Design review of the part built by this model. Coordinates are the model's own, in mm. A direction names the side the tool comes from. Coordinates: 2 decimals unless noted, no trailing zeros. Loops run counter-clockwise (first coordinate to the right, second up) from the corner with the lowest first, then second, coordinate; pieces in that order, holes last. Notation, with made-up numbers: (83, 30.25) -> (87, 30.25) arc R24 ccw to (87, 61.25) -> close; hole circle Ø9 at (24, -19). An arc over 180 degrees is marked (long way). Use CSV: the item, a comma, the result in double quotes.
```python
from build123d import *

# Parameters (mm, degrees)
SKETCH1_R           = 23
SKETCH1_R_2         = 0.725
BOSS_EXTRUDE1_DEPTH = 5
SKETCH2_W           = 4.5
SKETCH2_H           = 3.9
SKETCH2_W_2         = 3.9
SKETCH2_H_2         = 4.5
CUT_EXTRUDE1_DEPTH  = 6
SKETCH3_W           = 7
SKETCH3_H           = 4
SKETCH3_W_2         = 4
SKETCH3_H_2         = 7
CUT_EXTRUDE2_DEPTH  = 6


with BuildPart() as part:
    # Sketch1 → Boss-Extrude1 (new body)
    with BuildSketch(Plane.XY):
        Circle(SKETCH1_R)
        Circle(SKETCH1_R_2, mode=Mode.SUBTRACT)
    extrude(amount=BOSS_EXTRUDE1_DEPTH)

    # Sketch2 → Cut-Extrude1 (cut, through all)
    with BuildSketch(Plane(origin=(0, 0, 0), x_dir=(-1, 0, 0), z_dir=(0, 0, -1))):
        with Locations((9.999907629, 0.148804685)):
            Rectangle(SKETCH2_W, SKETCH2_H)
        with Locations((-0.147804685, 9.998907629)):
            Rectangle(SKETCH2_W_2, SKETCH2_H_2)
        with Locations((0.149804685, -9.998907629)):
            Rectangle(SKETCH2_W_2, SKETCH2_H_2)
        with Locations((-9.997907629, -0.148804685)):
            Rectangle(SKETCH2_W, SKETCH2_H)
    extrude(amount=-CUT_EXTRUDE1_DEPTH, mode=Mode.SUBTRACT)

    # Sketch3 → Cut-Extrude2 (cut, through all)
    with BuildSketch(Plane(origin=(0, 0, 0), x_dir=(-1, 0, 0), z_dir=(0, 0, -1))):
        with Locations((23, 0)):
            Rectangle(SKETCH3_W, SKETCH3_H)
        with Locations((0, 23)):
            Rectangle(SKETCH3_W_2, SKETCH3_H_2)
        with Locations((0, -23)):
            Rectangle(SKETCH3_W_2, SKETCH3_H_2)
        with Locations((-23, 0)):
            Rectangle(SKETCH3_W, SKETCH3_H)
    extrude(amount=-CUT_EXTRUDE2_DEPTH, mode=Mode.SUBTRACT)


solid = part.part
```
Item 1: Machinability: for faces 1 (the face through (-21, 2, 2)), 2 (the face through (12.248, 0, 2)), 3 (the face through (0, -19.5, 2)), which of the approach directions +Z, -Z, +X, -X, +Y, -Y give a long, thin tool a straight path to every point of the face, cutting with its end or side? Answer none if there is none.
Checked values:
face 1,"+Z, -Z, -X"
face 2,"+Z, -Z"
face 3,"+Z, -Z, -Y"
Item 2: Add section D-D (y = 8.5). Give the boundary of the cut face in (x, z).
Checked values:
outline,"(-21.37, 0) -> (-1.8, 0) -> (-1.8, 5) -> (-21.37, 5) -> close; (2.1, 0) -> (21.37, 0) -> (21.37, 5) -> (2.1, 5) -> close"
Item 3: Add section A-A (x = 0). Give the boundary of the cut face in (y, z) (3 decimals), then the cut area to 3 significant figures.
Checked values:
outline,"(-19.5, 0) -> (-12.249, 0) -> (-12.249, 5) -> (-19.5, 5) -> close; (-7.749, 0) -> (-0.725, 0) -> (-0.725, 5) -> (-7.749, 5) -> close; (0.725, 0) -> (7.749, 0) -> (7.749, 5) -> (0.725, 5) -> close; (12.249, 0) -> (19.5, 0) -> (19.5, 5) -> (12.249, 5) -> close"
area,"143 mm^2"
Item 4: Clearance check with flat-ended pins moving along their axes: pin 1 (1.3 mm diameter, centred on x = 11, z = 3.5, fed in from +Y); pin 2 (2.5 mm diameter, centred on y = -20.5, z = 3.5, fed in from -X); pin 3 (1 mm diameter, centred on y = -5, z = 0.5, fed in from -X). State where each tip first meets the part, or that it passes through.
Checked values:
pin 1,"y = 20.54"
pin 2,"x = -12.59"
pin 3,"x = -22.56"
Item 5: Add section B-B (y = 0). Give the boundary of the cut face in (x, z) (3 decimals).
Checked values:
outline,"(-19.5, 0) -> (-12.25, 0) -> (-12.25, 5) -> (-19.5, 5) -> close; (-7.75, 0) -> (-0.725, 0) -> (-0.725, 5) -> (-7.75, 5) -> close; (0.725, 0) -> (7.748, 0) -> (7.748, 5) -> (0.725, 5) -> close; (12.248, 0) -> (19.5, 0) -> (19.5, 5) -> (12.248, 5) -> close"
Item 6: Add section C-C (z = 3.1). State how many separate pieces and enclosed holes the cut face has, then the cut area to 3 significant figures.
Checked values:
separate pieces,"1"
enclosed holes,"5"
area,"1,530 mm^2"
Item 7: Draft analysis for pull direction Y (two halves, no side actions). For faces 4 (the face through (-2, -21, 2)), 5 (the face through (-0.724, 0.032, 2.465)), 6 (the face through (-16.104, 16.422, 2.465)), state which applies: pulls with the +Y half, pulls with the -Y half, needs draft (parallel to the pull), parting line crosses it, or undercut.
Checked values:
face 4,"needs draft"
face 5,"undercut"
face 6,"pulls with the +Y half"
Item 8: To check wall thickness, follow line 1 along Y through (x, z) = (0, 2.95) (3 decimals); line 2 along Y through (x, z) = (-1, 2.65); line 3 along X through (y, z) = (20, 3.05). State the ranges of each line that lie inside material, in increasing order.
Checked values:
line 1,"-19.5 to -12.249, -7.749 to -0.725, 0.725 to 7.749, 12.249 to 19.5"
line 2,"-19.5 to -12.25, -7.75 to 7.75, 12.25 to 19.5"
line 3,"-11.36 to -2, 2 to 11.36"
